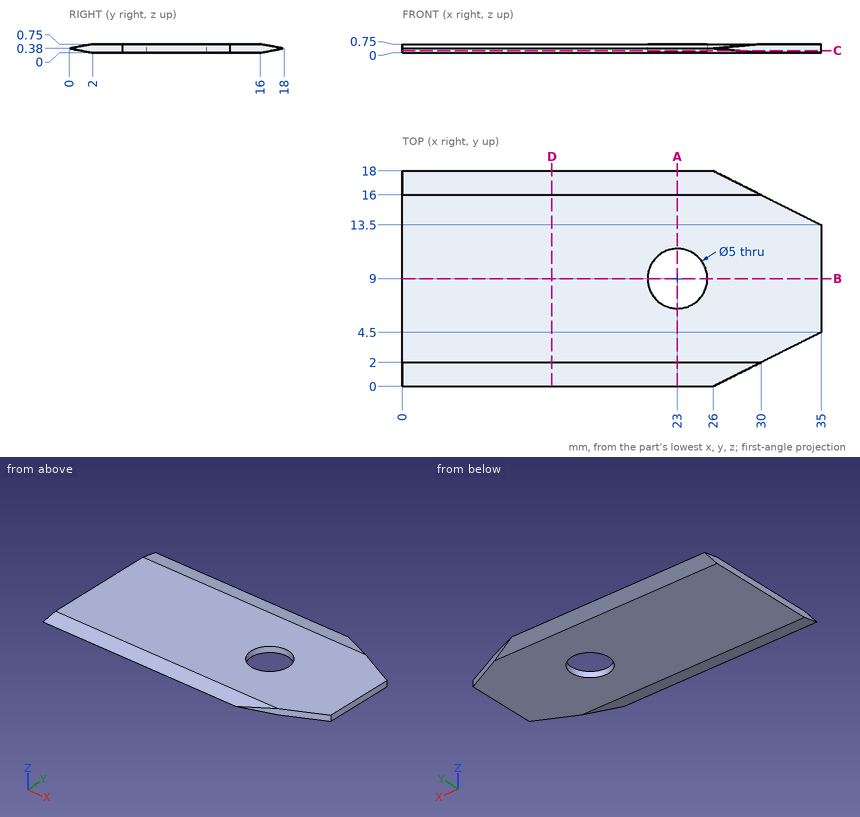
Check sheet for the drawn part. Datum: minimum x, y, z corner. Units: mm. Round coordinates to 2 decimals unless told otherwise and drop trailing zeros. Loops run counter-clockwise (first coordinate to the right, second up) from the corner with the lowest first, then second, coordinate; pieces in that order, holes last. Notation, with made-up numbers: M 29,63.5 L 72,63.5 A9 ccw 72,68.5 Z; hole C 89.25,67 d10. An arc over 180 degrees is marked long. Write each question's results on one line, items separated by ' | '.
1) Section check B-B on y = 9. Record the boundary of the cut face in (x, z).
Checks:
outline: M 0,0 L 20.5,0 L 20.5,0.75 L 0,0.75 Z; M 25.5,0 L 35,0 L 35,0.75 L 25.5,0.75 Z
2) Section check D-D on x = 12.5. Record the boundary of the cut face in (y, z), then the cut area to 3 significant figures.
Checks:
outline: M 0,0.38 L 2,0 L 16,0 L 18,0.38 L 16,0.75 L 2,0.75 Z | area: 12.0 mm2
3) Section check A-A on x = 23. Record the boundary of the cut face in (y, z), then the cut area to 3 significant figures.
Checks:
outline: M 0,0.38 L 2,0 L 6.5,0 L 6.5,0.75 L 2,0.75 Z; M 11.5,0 L 16,0 L 18,0.38 L 16,0.75 L 11.5,0.75 Z | area: 8.25 mm2
4) Gauge pin test, flat end, axial feed: P1, Ø4.5, axis at x = 23, y = 9, coming from the -Z side. Record the tip position at first contact, or that the pin passes through.
Checks:
P1: passes through
5) Section check C-C on z = 0.2. Record the boundary of the cut face in (x, y).
Checks:
outline: M 0,0.95 L 27.89,0.95 L 35,4.5 L 35,13.5 L 27.89,17.05 L 0,17.05 Z; hole C 23,9 d5
6) Scan lines: L1, parallel to Z at x = 19, y = 1.5 (1 decimal); L2, parallel to Z at x = 13.5, y = 17.25; L3, parallel to Y at x = 29.5, z = 0.4. Record each from-to range of solid material in increasing order. Write a range as from..to.
Checks:
L1: z = 0.1..0.7 | L2: z = 0.24..0.52 | L3: y = 1.75..16.25
